Work out the finished part from the listing and answer in its coordinate system (mm). Face numbers are marked on the shaded views. Round coordinates to 2 decimals unless told otherwise and drop trailing zeros. Loops run counter-clockwise (first coordinate to the right, second up) from the corner with the lowest first, then second, coordinate; pieces in that order, holes last.
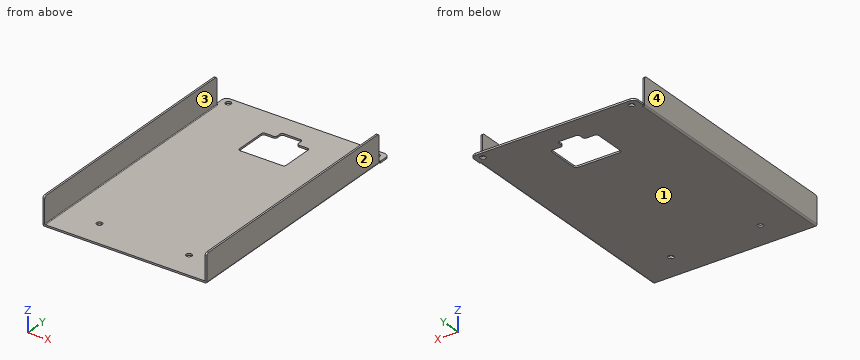
```python
from build123d import *

# Parameters (mm, degrees)
F1_R     = 1.2
F2_DEPTH = 0.744
F3_W     = 0.744
F3_H     = 103
F3_H_2   = 103.0000144269
F4_DEPTH = 12
F5_R     = 1
F6_W     = 0.744
F6_H     = 0.5
F7_DEPTH = 25
F8_R     = 0.3
F9_R     = 0.65
F10_R    = 0.3


# Not quite as in the source:
# - ends of sketch curves that miss each other by under 0.0002 mm in the source are joined


with BuildPart() as f2:
    # F1 (on Top) → F2 (new body)
    with BuildSketch(Plane.XY):
        with BuildLine():
            Line((-39.500012, -54.4999965731), (30.29995, -54.5000015731))
            Line((30.29995, -54.5000015731), (30.29995, 52.5000044269))
            ThreePointArc((30.29995, 52.5000044269), (29.7141635624, 53.9142179893), (28.29995, 54.5000044269))
            Line((28.29995, 54.5000044269), (-37.500012, 54.5000044269))
            ThreePointArc((-37.500012, 54.5000044269), (-38.9142255624, 53.9142179893), (-39.500012, 52.5000044269))
            Line((-39.500012, 52.5000044269), (-39.500012, -54.4999965731))
        make_face()
        with Locations((-23.649861, -42.9501055731)):
            Circle(F1_R, mode=Mode.SUBTRACT)
        with Locations((14.450063, -42.9501055731)):
            Circle(F1_R, mode=Mode.SUBTRACT)
        with Locations((-36.250012, 51.7500052865)):
            Circle(F1_R, mode=Mode.SUBTRACT)
        with BuildLine():
            Line((0.899969, 41.9500044269), (4.34995, 41.9500044269))
            ThreePointArc((4.34995, 41.9500044269), (5.0570567812, 41.6571112081), (5.34995, 40.9500044269))
            Line((5.34995, 40.9500044269), (5.34995, 27.9500044269))
            ThreePointArc((5.34995, 27.9500044269), (5.0570567812, 27.2428976457), (4.34995, 26.9500044269))
            Line((4.34995, 26.9500044269), (-13.55005, 26.9500044269))
            ThreePointArc((-13.55005, 26.9500044269), (-14.2571567812, 27.2428976457), (-14.55005, 27.9500044269))
            Line((-14.55005, 27.9500044269), (-14.55005, 40.9500044269))
            ThreePointArc((-14.55005, 40.9500044269), (-14.2571567812, 41.6571112081), (-13.55005, 41.9500044269))
            Line((-13.55005, 41.9500044269), (-10.100031, 41.9500044269))
            ThreePointArc((-10.100031, 41.9500044269), (-9.3929242188, 42.2428976457), (-9.100031, 42.9500044269))
            Line((-9.100031, 42.9500044269), (-9.100031, 44.4500044269))
            ThreePointArc((-9.100031, 44.4500044269), (-8.8071377812, 45.1571112081), (-8.100031, 45.4500044269))
            Line((-8.100031, 45.4500044269), (-4.600031, 45.4500044269))
            Line((-4.600031, 45.4500044269), (-1.100031, 45.4500044269))
            ThreePointArc((-1.100031, 45.4500044269), (-0.3929242188, 45.1571112081), (-0.100031, 44.4500044269))
            Line((-0.100031, 44.4500044269), (-0.100031, 42.9500044269))
            ThreePointArc((-0.100031, 42.9500044269), (0.1928622188, 42.2428976457), (0.899969, 41.9500044269))
        make_face(mode=Mode.SUBTRACT)
        with Locations((27.04995, 51.750023553)):
            Circle(F1_R, mode=Mode.SUBTRACT)
    extrude(amount=F2_DEPTH)

    # F3 (on face) → F4 (join)
    with BuildSketch(Plane(origin=(0, 0, 0), x_dir=(1, 0, 0), z_dir=(0, 0, -1))):
        with Locations((29.92795, 2.9999821461)):
            Rectangle(F3_W, F3_H)
        with Locations((-39.128012, 2.9999893596)):
            Rectangle(F3_W, F3_H_2)
    extrude(amount=-F4_DEPTH)

    # F5
    f5_edges = [f2.edges().sort_by_distance(p)[0] for p in [
        (29.92795, -54.499982, 12),
        (29.92795, 48.500018, 12),
        (-39.128012, 48.500018, 12),
        (-39.128012, -54.499997, 12),
    ]]
    fillet(f5_edges, radius=F5_R)

    # F6 (on face) → F7 (cut)
    with BuildSketch(Plane.XY.offset(0.744)):
        with Locations((-39.128012, 48.7500178539)):
            Rectangle(F6_W, F6_H)
        with Locations((29.92795, 48.7500178539)):
            Rectangle(F6_W, F6_H)
    extrude(amount=-F7_DEPTH, mode=Mode.SUBTRACT)

    # F8
    f8_edges = [f2.edges().sort_by_distance(p)[0] for p in [
        (30.29995, 49.000018, 0.372),
        (29.55595, 49.000018, 0.372),
        (-39.500012, 49.000018, 0.372),
        (-38.756012, 49.000018, 0.372),
    ]]
    fillet(f8_edges, radius=F8_R)

    # F9
    f9_edges = [f2.edges().sort_by_distance(p)[0] for p in [
        (-39.500012, -2.999989, 0),
        (30.29995, -2.999992, 0),
    ]]
    fillet(f9_edges, radius=F9_R)

    # F10
    f10_edges = [f2.edges().sort_by_distance(p)[0] for p in [
        (-38.756012, -2.999989, 0.744),
        (29.55595, -2.999982, 0.744),
    ]]
    fillet(f10_edges, radius=F10_R)


solid = f2.part
```
1. Find section A-A (y = 39.5). Write down the section's boundary in (x, z).
Answer key:
outline: (-39.5, 0.65) arc R0.65 ccw to (-38.85, 0) - (-14.55, 0) - (-14.55, 0.74) - (-38.46, 0.74) arc R0.3 cw to (-38.76, 1.04) - (-38.76, 12) - (-39.5, 12) - close; (5.35, 0) - (29.65, 0) arc R0.65 ccw to (30.3, 0.65) - (30.3, 12) - (29.56, 12) - (29.56, 1.04) arc R0.3 cw to (29.26, 0.74) - (5.35, 0.74) - close
2. Find section B-B (x = -7). Write down the section's boundary in (y, z).
Answer key:
outline: (-54.5, 0) - (26.95, 0) - (26.95, 0.74) - (-54.5, 0.74) - close; (45.45, 0) - (54.5, 0) - (54.5, 0.74) - (45.45, 0.74) - close
3. Given pin 1 (2 mm diameter, centred on x = 14.45, y = -42.95, fed in from -Z); pin 2 (0.5 mm diameter, centred on x = -39, z = 6, fed in from +Y); pin 3 (1 mm diameter, centred on x = 17.5, y = -35.5, fed in from +Z), each flat-ended and moving along its own axis, determine where each tip first touches the part or whether it passes through.
Answer key:
pin 1: passes through
pin 2: stops at y = 48.5
pin 3: stops at z = 0.74
4. Find section C-C (z = 7.75). Write down the section's boundary in (x, y).
Answer key:
outline: (-39.5, -54.5) - (-38.76, -54.5) - (-38.76, 48.5) - (-39.5, 48.5) - close; (29.56, -54.5) - (30.3, -54.5) - (30.3, 48.5) - (29.56, 48.5) - close
5. Consider probe 1 along X at (y, z) = (-45.5, 1.25); probe 2 along Z at (x, y) = (-6, -49). Determine where each line is inside the solid, lowest interval first.
Answer key:
probe 1: x = -39.5 to -38.76, 29.56 to 30.3
probe 2: z = 0 to 0.74
6. Find section D-D (y = -36). Write down the section's boundary in (x, z).
Answer key:
outline: (-39.5, 0.65) arc R0.65 ccw to (-38.85, 0) - (29.65, 0) arc R0.65 ccw to (30.3, 0.65) - (30.3, 12) - (29.56, 12) - (29.56, 1.04) arc R0.3 cw to (29.26, 0.74) - (-38.46, 0.74) arc R0.3 cw to (-38.76, 1.04) - (-38.76, 12) - (-39.5, 12) - close
7. Determine the mould class of the marked faces 1, 2, 3 and 4 for opening direction X: +X half, -X half, draft (parallel to the pull), parting line (faces both ways), or undercut.
Answer key:
face 1: draft
face 2: +X half
face 3: undercut
face 4: -X half
